For this review, take the finished solid that the model builds, in its own axes (mm). A direction names the side the tool comes from. Give positions to 0.01 mm unless a question says otherwise; leave off trailing zeros. Loops run counter-clockwise (first coordinate to the right, second up) from the corner with the lowest first, then second, coordinate; pieces in that order, holes last.
```python
from build123d import *

# Parameters (mm, degrees)
ESQUISSE1_R        = 1.75
ESQUISSE1_R_2      = 10.25
BOSS_EXTRU_1_DEPTH = 6
CONG_1_R           = 4
CONG_2_R           = 1.5


with BuildPart() as part:
    # Esquisse1 → Boss.-Extru.1 (new body)
    with BuildSketch(Plane.XY):
        with BuildLine():
            Line((117, -130), (127.5, -130))
            Line((127.5, -130), (127.5, 130))
            Line((127.5, 130), (117, 130))
            Line((117, 130), (117, 109))
            Line((117, 109), (110.199818512, 109))
            ThreePointArc((110.199818512, 109), (105.313920853, 107.562324439), (101.985331022, 103.707535642))
            ThreePointArc((101.985331022, 103.707535642), (0, 38), (-101.985331022, 103.707535642))
            ThreePointArc((-101.985331022, 103.707535642), (-105.313920853, 107.562324439), (-110.199818512, 109))
            Line((-110.199818512, 109), (-117, 109))
            Line((-117, 109), (-117, 130))
            Line((-117, 130), (-127.5, 130))
            Line((-127.5, 130), (-127.5, -130))
            Line((-127.5, -130), (-117, -130))
            Line((-117, -130), (-117, -109))
            Line((-117, -109), (-110.199818512, -109))
            ThreePointArc((-110.199818512, -109), (-105.313920853, -107.562324439), (-101.985331022, -103.707535642))
            ThreePointArc((-101.985331022, -103.707535642), (0, -38), (101.985331022, -103.707535642))
            ThreePointArc((101.985331022, -103.707535642), (105.313920853, -107.562324439), (110.199818512, -109))
            Line((110.199818512, -109), (117, -109))
            Line((117, -109), (117, -130))
        make_face()
        with Locations((-123.5, -123.75)):
            Circle(ESQUISSE1_R, mode=Mode.SUBTRACT)
        with Locations((-123.5, -111.25)):
            Circle(ESQUISSE1_R, mode=Mode.SUBTRACT)
        with Locations((-123.5, -105)):
            Circle(ESQUISSE1_R, mode=Mode.SUBTRACT)
        with Locations((-112, -93.5)):
            Circle(ESQUISSE1_R_2, mode=Mode.SUBTRACT)
        with Locations((-123.5, -82)):
            Circle(ESQUISSE1_R, mode=Mode.SUBTRACT)
        with Locations((-100.5, -82)):
            Circle(ESQUISSE1_R, mode=Mode.SUBTRACT)
        with Locations((-109, -70)):
            Circle(ESQUISSE1_R, mode=Mode.SUBTRACT)
        with Locations((-109, -55)):
            Circle(ESQUISSE1_R, mode=Mode.SUBTRACT)
        with Locations((-36.3, -20)):
            Circle(ESQUISSE1_R, mode=Mode.SUBTRACT)
        with Locations((-16.3, -20)):
            Circle(ESQUISSE1_R, mode=Mode.SUBTRACT)
        with Locations((123.5, -123.75)):
            Circle(ESQUISSE1_R, mode=Mode.SUBTRACT)
        with Locations((123.5, -111.25)):
            Circle(ESQUISSE1_R, mode=Mode.SUBTRACT)
        with Locations((123.5, -105)):
            Circle(ESQUISSE1_R, mode=Mode.SUBTRACT)
        with Locations((100.5, -82)):
            Circle(ESQUISSE1_R, mode=Mode.SUBTRACT)
        with Locations((112, -93.5)):
            Circle(ESQUISSE1_R_2, mode=Mode.SUBTRACT)
        with Locations((123.5, -82)):
            Circle(ESQUISSE1_R, mode=Mode.SUBTRACT)
        with Locations((109, -70)):
            Circle(ESQUISSE1_R, mode=Mode.SUBTRACT)
        with Locations((0, -35)):
            Circle(ESQUISSE1_R, mode=Mode.SUBTRACT)
        with Locations((0, -16.5)):
            Circle(ESQUISSE1_R, mode=Mode.SUBTRACT)
        with Locations((16.3, -20)):
            Circle(ESQUISSE1_R, mode=Mode.SUBTRACT)
        with Locations((36.3, -20)):
            Circle(ESQUISSE1_R, mode=Mode.SUBTRACT)
        with Locations((109, -55)):
            Circle(ESQUISSE1_R, mode=Mode.SUBTRACT)
        Polygon((-89.5, 38), (-41.5, 38), (-41.5, -38), (-89.5, -38), (-89.5, -41.5), (-124.5, -41.5), (-124.5, 41.5), (-89.5, 41.5), align=None, mode=Mode.SUBTRACT)
        with Locations((-109, 55)):
            Circle(ESQUISSE1_R, mode=Mode.SUBTRACT)
        with Locations((-36.3, 20)):
            Circle(ESQUISSE1_R, mode=Mode.SUBTRACT)
        with Locations((-16.3, 20)):
            Circle(ESQUISSE1_R, mode=Mode.SUBTRACT)
        with Locations((0, 35)):
            Circle(ESQUISSE1_R, mode=Mode.SUBTRACT)
        with Locations((-109, 70)):
            Circle(ESQUISSE1_R, mode=Mode.SUBTRACT)
        with Locations((-123.5, 82)):
            Circle(ESQUISSE1_R, mode=Mode.SUBTRACT)
        with Locations((-112, 93.5)):
            Circle(ESQUISSE1_R_2, mode=Mode.SUBTRACT)
        with Locations((-100.5, 82)):
            Circle(ESQUISSE1_R, mode=Mode.SUBTRACT)
        with Locations((-123.5, 105)):
            Circle(ESQUISSE1_R, mode=Mode.SUBTRACT)
        with Locations((-123.5, 111.25)):
            Circle(ESQUISSE1_R, mode=Mode.SUBTRACT)
        with Locations((-123.5, 123.75)):
            Circle(ESQUISSE1_R, mode=Mode.SUBTRACT)
        with Locations((0, 16.5)):
            Circle(ESQUISSE1_R, mode=Mode.SUBTRACT)
        with Locations((16.3, 20)):
            Circle(ESQUISSE1_R, mode=Mode.SUBTRACT)
        with Locations((36.3, 20)):
            Circle(ESQUISSE1_R, mode=Mode.SUBTRACT)
        Polygon((41.5, 38), (89.5, 38), (89.5, 41.5), (124.5, 41.5), (124.5, -41.5), (89.5, -41.5), (89.5, -38), (41.5, -38), align=None, mode=Mode.SUBTRACT)
        with Locations((109, 55)):
            Circle(ESQUISSE1_R, mode=Mode.SUBTRACT)
        with Locations((109, 70)):
            Circle(ESQUISSE1_R, mode=Mode.SUBTRACT)
        with Locations((100.5, 82)):
            Circle(ESQUISSE1_R, mode=Mode.SUBTRACT)
        with Locations((123.5, 82)):
            Circle(ESQUISSE1_R, mode=Mode.SUBTRACT)
        with Locations((112, 93.5)):
            Circle(ESQUISSE1_R_2, mode=Mode.SUBTRACT)
        with Locations((123.5, 105)):
            Circle(ESQUISSE1_R, mode=Mode.SUBTRACT)
        with Locations((123.5, 111.25)):
            Circle(ESQUISSE1_R, mode=Mode.SUBTRACT)
        with Locations((123.5, 123.75)):
            Circle(ESQUISSE1_R, mode=Mode.SUBTRACT)
    extrude(amount=BOSS_EXTRU_1_DEPTH)

    # Congé1
    cong_1_edges = [part.edges().sort_by_distance(p)[0] for p in [
        (-117, -109, 3),
        (-117, -130, 3),
        (-127.5, -130, 3),
        (-127.5, 130, 3),
        (-117, 130, 3),
        (-117, 109, 3),
        (117, 109, 3),
        (117, 130, 3),
        (127.5, 130, 3),
        (127.5, -130, 3),
        (117, -130, 3),
        (117, -109, 3),
    ]]
    fillet(cong_1_edges, radius=CONG_1_R)

    # Congé2
    cong_2_edges = [part.edges().sort_by_distance(p)[0] for p in [
        (41.5, -38, 3),
        (89.5, -38, 3),
        (89.5, -41.5, 3),
        (124.5, -41.5, 3),
        (124.5, 41.5, 3),
        (89.5, 41.5, 3),
        (89.5, 38, 3),
        (41.5, 38, 3),
        (-89.5, 41.5, 3),
        (-124.5, 41.5, 3),
        (-124.5, -41.5, 3),
        (-89.5, -41.5, 3),
        (-89.5, -38, 3),
        (-41.5, -38, 3),
        (-41.5, 38, 3),
        (-89.5, 38, 3),
    ]]
    fillet(cong_2_edges, radius=CONG_2_R)


solid = part.part
```
Q1. Mouldability with a two-part tool opening along Y and no side actions: class faces 5 (the cylindrical face through (1.795, 38.014, 2.958)), 6 (the flat face through (-127.5, 2, 3)), 7 (the cylindrical face through (-102.223, 96.579, 2.958)) as +Y half, -Y half, draft (parallel to the pull), parting line (faces both ways), or undercut.
Answers:
face 5: +Y half
face 6: draft
face 7: undercut
Q2. Machinability: for faces 1 (the flat face through (65, 38, 3)), 2 (the flat face through (127.5, -2, 3)), 3 (the flat face through (117, 120, 3)), 4 (the flat face through (-117, -120, 3)), which of the approach directions +Z, -Z, +X, -X, +Y, -Y give a long, thin tool a straight path to every point of the face, cutting with its end or side? Answer none if there is none.
Answers:
face 1: +Z, -Z
face 2: +Z, -Z, +X, +Y, -Y
face 3: +Z, -Z, +Y
face 4: +Z, -Z, -Y
Q3. For probe 1 along X at (y, z) = (-10.5, 4.4); probe 2 along Y at (x, z) = (115, 2.65); probe 3 along X at (y, z) = (-82, 2.95), list the stretches that pass through material, from the lowest coordinate up.
Answers:
probe 1: x = -127.5 to -124.5, -41.5 to 41.5, 124.5 to 127.5
probe 2: y = -109.54 to -103.3, -83.7 to -41.5, 41.5 to 83.7, 103.3 to 109.54
probe 3: x = -127.5 to -125.25, -121.75 to -102.25, -98.75 to -88.99, 88.99 to 98.75, 102.25 to 121.75, 125.25 to 127.5
Q4. Consider section C-C on y = 49. Give the boundary of the cut face in (x, z), plus the area to 3 significant figures.
Answers:
outline: (-127.5, 0) - (-48.4, 0) - (-48.4, 6) - (-127.5, 6) - close; (48.4, 0) - (127.5, 0) - (127.5, 6) - (48.4, 6) - close
area: 949 mm2
Q5. Consider section A-A on y = 4. Give the boundary of the cut face in (x, z).
Answers:
outline: (-127.5, 0) - (-124.5, 0) - (-124.5, 6) - (-127.5, 6) - close; (-41.5, 0) - (41.5, 0) - (41.5, 6) - (-41.5, 6) - close; (124.5, 0) - (127.5, 0) - (127.5, 6) - (124.5, 6) - close
Q6. Consider section D-D on y = 93.5. Give the boundary of the cut face in (x, z), plus the area to 3 significant figures.
Answers:
outline: (-127.5, 0) - (-122.25, 0) - (-122.25, 6) - (-127.5, 6) - close; (-101.75, 0) - (-96.7, 0) - (-96.7, 6) - (-101.75, 6) - close; (96.7, 0) - (101.75, 0) - (101.75, 6) - (96.7, 6) - close; (122.25, 0) - (127.5, 0) - (127.5, 6) - (122.25, 6) - close
area: 124 mm2
Q7. For pin 1 Ø1.5 at (x, z) = (8, 3) entering from +Y; pin 2 Ø3 at (x, z) = (-111.5, 4.5) entering from +Y, all flat-tipped, find the tip position at first contact; note any pin that passes through.
Answers:
pin 1: stops at y = 38.34
pin 2: stops at y = 109
Q8. Consider section B-B on z = 4.2. Count the separate pieces of the cut face and the enclosed holes in it, plus the area to 3 significant figures.
Answers:
separate pieces: 1
enclosed holes: 46
area: 20,200 mm2
